Verification items for the finished model (mm, model axes). A direction names the side the tool comes from. Round coordinates to 2 decimals unless told otherwise and drop trailing zeros. Write each loop counter-clockwise with the first axis right and the second up, starting at its lowest first coordinate (ties: lowest second). Pieces come first, ordered by that corner, then holes. Notation, with made-up numbers: (20.25, 66) -> (58.25, 66) arc R18 cw to (58.25, 94) -> close; hole circle Ø11 at (76.25, 19). An arc over 180 degrees is marked (long way). Answer as a JSON object with one key per item and string values. Group by question number.
(1) Sectioned sample at D-D on z = -7.5. Record the cut outline in (x, y), and give its area (3 significant figures).
(2) Scan lines: L1, parallel to Y at x = -44, z = -18.5; L2, parallel to X at y = 3.7, z = 25.5; L3, parallel to X at y = 1.3, z = 25.5. Record each from-to range of solid material in increasing order. Write a range as from..to.
(3) Sectioned sample at C-C on y = 8. Record the cut outline in (x, z).
(4) Gauge pin test, flat ends, axial feed: pin 1 Ø0.8 at (x, z) = (-33, -10.5) entering from +Y; pin 2 Ø3 at (y, z) = (3, 14) entering from -X; pin 3 Ø1.5 at (x, z) = (-43, -25) entering from -Y. Record the tip position at first contact, or that the pin passes through.
(5) Sectioned sample at A-A on z = -27. Record the cut outline in (x, y), and give its area (3 significant figures).
(6) Set-up check for faces 4 (the face through (-45.44, 2.96, 26.04)), 5 (the face through (48.4, 24.43, -0.41)), 6 (the face through (-52, 18, 14)), 7 (the face through (-44, 14, -2.907)): record each of +Z, -Z, +X, -X, +Y, -Y from which the full face is reachable in a straight line by a thin tool's end or side.
(7) Draft check along Y on faces 1 (the face through (-44, 21, -6)), 2 (the face through (40.56, 2.96, -24.96)), 3 (the face through (-52, 12, 14)). Enter one of: released by +Y, released by -Y, zero draft, split by the parting line, or undercut.
(8) Sectioned sample at B-B on x = -44. Record the cut outline in (y, z), and give its area (3 significant figures).
```python
from build123d import *

# Parameters (mm, degrees)
SKETCH2_W           = 98
SKETCH2_H           = 62
BOSS_EXTRUDE1_DEPTH = 25
SKETCH3_W           = 9.5
SKETCH3_H           = 12
BOSS_EXTRUDE4_DEPTH = 1
SKETCH3_5_W         = 9.5
SKETCH3_5_H         = 12
CUT_EXTRUDE1_DEPTH  = 1
SKETCH4_R           = 3.25
CUT_EXTRUDE2_DEPTH  = 10
SKETCH5_R           = 0.5
BOSS_EXTRUDE5_DEPTH = 8
SKETCH6_W           = 7
SKETCH6_H           = 14
CUT_EXTRUDE9_DEPTH  = 10
SKETCH7_W           = 1.559437484
SKETCH7_H           = 10
BOSS_EXTRUDE6_DEPTH = 9
SKETCH8_W           = 15
SKETCH8_H           = 10
BOSS_EXTRUDE7_DEPTH = 2
BOSS_EXTRUDE7_TAPER = 30
BOSS_EXTRUDE8_DEPTH = 6
FILLET5_R           = 2
SKETCH10_R          = 2.5
CUT_EXTRUDE10_DEPTH = 6
SKETCH11_R          = 0.5
CUT_EXTRUDE11_DEPTH = 3


with BuildPart() as part:
    # Sketch2 → Boss-Extrude1 (new body)
    with BuildSketch(Plane(origin=(0, 0, 0), x_dir=(1, 0, 0), z_dir=(0, 1, 0))):
        Rectangle(SKETCH2_W, SKETCH2_H)
    extrude(amount=BOSS_EXTRUDE1_DEPTH)

    # Sketch3 → Boss-Extrude4 (add)
    with BuildSketch(Plane.ZY.offset(49)):
        with Locations((-18.656971736, 15)):
            Rectangle(SKETCH3_W, SKETCH3_H)
    extrude(amount=-BOSS_EXTRUDE4_DEPTH)

    # Sketch3<5> → Cut-Extrude1 (cut)
    with BuildSketch(Plane.ZY.offset(49)):
        with Locations((-18.656971736, 15)):
            Rectangle(SKETCH3_5_W, SKETCH3_5_H)
    extrude(amount=-CUT_EXTRUDE1_DEPTH, mode=Mode.SUBTRACT)

    # Sketch4 → Cut-Extrude2 (cut)
    with BuildSketch(Plane.ZY.offset(48)):
        with Locations((-18.406971736, 16)):
            Circle(SKETCH4_R)
    extrude(amount=-CUT_EXTRUDE2_DEPTH, mode=Mode.SUBTRACT)

    # Sketch5 → Boss-Extrude5 (add)
    with BuildSketch(Plane.ZY.offset(38)):
        with Locations((-18.406971736, 16)):
            Circle(SKETCH5_R)
    extrude(amount=BOSS_EXTRUDE5_DEPTH)

    # Sketch6 → Cut-Extrude9 (cut)
    with BuildSketch(Plane.ZY.offset(49)):
        with Locations((-6.406971736, 14)):
            Rectangle(SKETCH6_W, SKETCH6_H)
    extrude(amount=-CUT_EXTRUDE9_DEPTH, mode=Mode.SUBTRACT)

    # Sketch7 → Boss-Extrude6 (add)
    with BuildSketch(Plane.ZY.offset(39)):
        with Locations((-4.686690478, 14)):
            Rectangle(SKETCH7_W, SKETCH7_H)
    extrude(amount=BOSS_EXTRUDE6_DEPTH)

    # Sketch8 → Boss-Extrude7 (add)
    with BuildSketch(Plane.ZY.offset(49)):
        with Locations((12.093028264, 15)):
            Rectangle(SKETCH8_W, SKETCH8_H)
    extrude(amount=BOSS_EXTRUDE7_DEPTH, taper=BOSS_EXTRUDE7_TAPER)

    # Sketch9 → Boss-Extrude8 (add)
    with BuildSketch(Plane(origin=(0, 12, 0), x_dir=(-1, 0, 0), z_dir=(0, -1, 0))):
        with BuildLine():
            Line((51, -7.644654734), (51, -16.805465041))
            add(Edge.make_bspline(
                [(53.813384295, -15.000246539), (53.104445278, -16.821688465), (51, -16.805465041)],
                knots=[0, 0, 0, 1, 1, 1], degree=2))
            add(Edge.make_bspline(
                [(51, -7.644654734), (51.419023322, -11.667929153), (53.813384295, -15.000246539)],
                knots=[0, 0, 0, 1, 1, 1], degree=2))
        make_face()
    extrude(amount=-BOSS_EXTRUDE8_DEPTH)

    # Fillet5
    fillet5_edges = [part.edges().sort_by_distance(p)[0] for p in [
        (0, 25, 31),
        (-49, 25, 0),
        (0, 25, -31),
        (-49, 0, 0),
        (0, 0, 31),
        (49, 0, 0),
        (0, 0, -31),
        (49, 25, 0),
        (-49, 12.5, -31),
        (-49, 12.5, 31),
        (49, 12.5, 31),
        (49, 12.5, -31),
    ]]
    fillet(fillet5_edges, radius=FILLET5_R)

    # Sketch10 → Cut-Extrude10 (cut)
    with BuildSketch(Plane.XZ):
        with Locations(Location((-43, -25.5, 0), (0, 0, 270))):
            Circle(SKETCH10_R)
        with Locations(Location((-43, 25.5, 0), (0, 0, 270))):
            Circle(SKETCH10_R)
        with Locations(Location((43, 25.5, 0), (0, 0, 270))):
            Circle(SKETCH10_R)
        with Locations(Location((43, -25.5, 0), (0, 0, 270))):
            Circle(SKETCH10_R)
    extrude(amount=-CUT_EXTRUDE10_DEPTH, mode=Mode.SUBTRACT)

    # Sketch11 → Cut-Extrude11 (cut)
    with BuildSketch(Plane(origin=(0, 25, 0), x_dir=(1, 0, 0), z_dir=(0, 1, 0))):
        with Locations(Location((-33, 16.5, 0), (0, 0, 270))):
            Circle(SKETCH11_R)
        with Locations(Location((-33, 10.5, 0), (0, 0, 270))):
            Circle(SKETCH11_R)
        with Locations(Location((-33, 4.5, 0), (0, 0, 270))):
            Circle(SKETCH11_R)
        with Locations(Location((-33, -1.5, 0), (0, 0, 270))):
            Circle(SKETCH11_R)
        with Locations(Location((-33, -7.5, 0), (0, 0, 270))):
            Circle(SKETCH11_R)
    extrude(amount=-CUT_EXTRUDE11_DEPTH, mode=Mode.SUBTRACT)


solid = part.part
```
Computed values:
{
 "1": {"outline": "(-49, 2) arc R2 ccw to (-47, 0) -> (47, 0) arc R2 ccw to (49, 2) -> (49, 23) arc R2 ccw to (47, 25) -> (-47, 25) arc R2 ccw to (-49, 23) -> (-49, 21) -> (-39, 21) -> (-39, 7) -> (-49, 7) -> close", "area": "2,310 mm2"},
 "2": {"L1": "0..12.75, 15.51..16.49, 19.25..25", "L2": "-49..-45.5, -40.5..40.5, 45.5..49", "L3": "-48.87..-45.5, -40.5..40.5, 45.5..48.87"},
 "3": {"outline": "(-49, -29) arc R2 ccw to (-47, -31) -> (47, -31) arc R2 ccw to (49, -29) -> (49, 29) arc R2 ccw to (47, 31) -> (-47, 31) arc R2 ccw to (-49, 29) -> (-49, -2.91) -> (-39, -2.91) -> (-39, -9.91) -> (-49, -9.91) -> close"},
 "4": {"pin 1": "y = 22", "pin 2": "x = -49", "pin 3": "y = 6"},
 "5": {"outline": "(-49, 2) arc R2 ccw to (-47, 0) -> (-45, 0) -> (-45, 6) -> (-41, 6) -> (-41, 0) -> (41, 0) -> (41, 6) -> (45, 6) -> (45, 0) -> (47, 0) arc R2 ccw to (49, 2) -> (49, 23) arc R2 ccw to (47, 25) -> (-47, 25) arc R2 ccw to (-49, 23) -> close", "area": "2,400 mm2"},
 "6": {"face 4": "-Y", "face 5": "+Z, -Z, +X, +Y", "face 6": "+Z, -Z, -X, +Y", "face 7": "-X"},
 "7": {"face 1": "undercut", "face 2": "zero draft", "face 3": "released by -Y"},
 "8": {"outline": "(0, -29) arc R2 ccw to (2, -31) -> (23, -31) arc R2 ccw to (25, -29) -> (25, 29) arc R2 ccw to (23, 31) -> (2, 31) arc R2 ccw to (0, 29) -> (0, 27.79) -> (6, 27.79) -> (6, 23.21) -> (0, 23.21) -> (0, -23.21) -> (6, -23.21) -> (6, -27.79) -> (0, -27.79) -> close; (9, -5.47) -> (19, -5.47) -> (19, -3.91) -> (9, -3.91) -> close; circle Ø1 at (16, -18.41); hole (7, -9.91) -> (21, -9.91) -> (21, -2.91) -> (7, -2.91) -> close; hole circle Ø6.5 at (16, -18.41)", "area": "1,380 mm2"}
}
